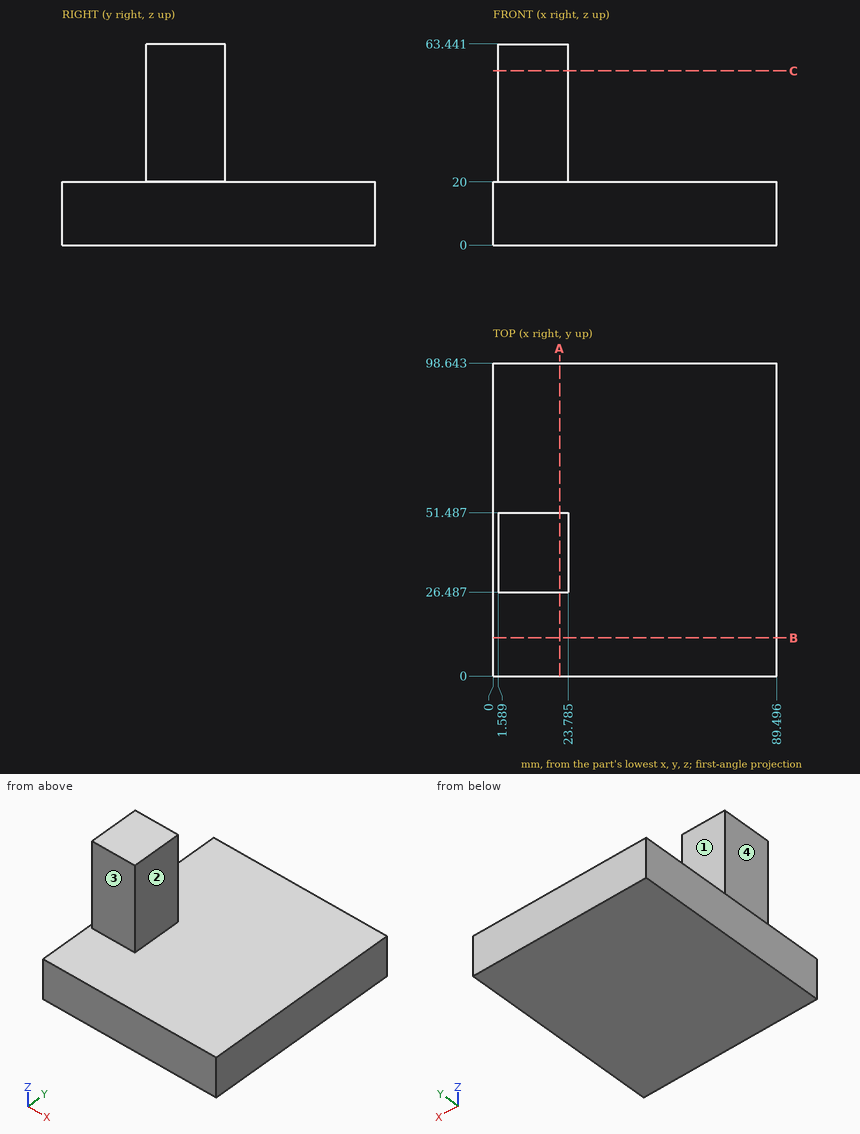
For this review, use the dimensioned drawing (mm, ordinates from the lowest corner) and the shaded views. A direction names the side the tool comes from. Round coordinates to 2 decimals unless told otherwise and drop trailing zeros. Write each loop counter-clockwise with the first axis right and the second up, starting at its lowest first coordinate (ties: lowest second). Pieces come first, ordered by that corner, then holes. Notation, with made-up numbers: (54, 77.25) - (82, 77.25) arc R18 ccw to (82, 94.25) - close; hole circle Ø1 at (-39, -31.5). An arc over 180 degrees is marked (long way). One line per item, written item: value. Start each with the question number.
1. Consider section C-C on z = 55. Write out the cut boundary in (x, y) (1 decimal).
2. Machinability: for the marked faces 1, 2, 3 and 4, which of the approach directions +Z, -Z, +X, -X, +Y, -Y give a long, thin tool a straight path to every point of the face, cutting with its end or side? Answer none if there is none.
3. Consider section A-A on x = 21. Write out the cut boundary in (y, z), and give its area (3 significant figures).
4. To check wall thickness, follow L1, parallel to Y at x = 14, z = 59.5; L2, parallel to Z at x = 41, y = 91; L3, parallel to X at y = 44, z = 25.5 (1 decimal). State the ranges of each line that lie inside material, in increasing order. Write a range as from..to.
5. Clearance check with flat-ended pins moving along their axes: P1, Ø12, axis at y = 53, z = 28, coming from the +X side (1 decimal); P2, Ø12.5, axis at y = 41.5, z = 46, coming from the -X side; P3, Ø12, axis at y = 77, z = 30, coming from the +X side; P4, Ø11, axis at x = 18, z = 32, coming from the -Y side. State where each tip first meets the part, or that it passes through.
6. Consider section B-B on y = 12. Write out the cut boundary in (x, z).
Checks:
1. outline: (1.6, 26.5) - (23.8, 26.5) - (23.8, 51.5) - (1.6, 51.5) - close
2. face 1: +Z, +X, -X, +Y
2. face 2: +Z, +X, +Y, -Y
2. face 3: +Z, +X, -X, -Y
2. face 4: +Z, -X, +Y, -Y
3. outline: (0, 0) - (98.64, 0) - (98.64, 20) - (51.49, 20) - (51.49, 63.44) - (26.49, 63.44) - (26.49, 20) - (0, 20) - close
3. area: 3,060 mm^2
4. L1: y = 26.49..51.49
4. L2: z = 0..20
4. L3: x = 1.6..23.8
5. P1: stops at x = 23.8
5. P2: stops at x = 1.59
5. P3: passes through
5. P4: stops at y = 26.49
6. outline: (0, 0) - (89.5, 0) - (89.5, 20) - (0, 20) - close
